from build123d import *

# Parameters (mm, degrees)
F1_DEPTH = 16
F2_W     = 7.5
F2_H     = 58


with BuildPart() as f1:
    # F0 (on Top) → F1 (new body)
    with BuildSketch(Plane.XY):
        with BuildLine():
            Line((-4.2, -8.4), (4.2, -8.4))
            ThreePointArc((4.2, -8.4), (7.028427, -7.228427), (8.2, -4.4))
            Line((8.2, -4.4), (8.2, 4.4))
            ThreePointArc((8.2, 4.4), (7.028427, 7.228427), (4.2, 8.4))
            Line((4.2, 8.4), (-4.2, 8.4))
            ThreePointArc((-4.2, 8.4), (-7.028427, 7.228427), (-8.2, 4.4))
            Line((-8.2, 4.4), (-8.2, -4.4))
            ThreePointArc((-8.2, -4.4), (-7.028427, -7.228427), (-4.2, -8.4))
        make_face()
    extrude(amount=-F1_DEPTH)

    # F2 (on Right) → F3 (revolve)
    with BuildSketch(Plane.YZ):
        Polygon((-10, 0), (0, 0), (0, 1.5), (-7.5, 1.5), (-10, 1.5), align=None)
        with Locations((-3.75, 30.5)):
            Rectangle(F2_W, F2_H)
        Polygon((-7.5, 59.5), (0, 59.5), (0, 60.5), (-8, 60.5), (-8, 59.5), align=None)
    revolve(axis=Axis((0, 0, 30.5), (0, 0, 1)))


solid = f1.part
Source: CAD feature listing. Evaluate the final solid. Frame: model axes, mm. A direction names the side the tool comes from. Coordinates: 2 decimals unless noted, no trailing zeros. Loops run counter-clockwise (first coordinate to the right, second up) from the corner with the lowest first, then second, coordinate; pieces in that order, holes last. Notation, with made-up numbers: M 73.5,34.25 L 113.5,34.25 A27 ccw 113.5,50.25 Z; hole C -25,16 d2. An arc over 180 degrees is marked long. Answer in a Markdown table with one row per item.
Q1. Section B-B on y = 0. Return the cut outline in (x, z), plus the area to 3 significant figures.
Answers below:
| item | result |
|---|---|
| outline | M -10,0 L -8.2,0 L -8.2,-16 L 8.2,-16 L 8.2,0 L 10,0 L 10,1.5 L 7.5,1.5 L 7.5,59.5 L 8,59.5 L 8,60.5 L -8,60.5 L -8,59.5 L -7.5,59.5 L -7.5,1.5 L -10,1.5 Z |
| area | 1,180 mm^2 |
Q2. Draft query along Z for faces 1 (the flat face through (-6, -5, 59.5)), 2 (the flat face through (9, 0, 0)), 3 (the flat face through (0, 0, 60.5)). Return one class per face: pulls with the +Z half, pulls with the -Z half, needs draft (parallel to the pull), parting line crosses it, or undercut.
Answers below:
| item | result |
|---|---|
| face 1 | undercut |
| face 2 | pulls with the -Z half |
| face 3 | pulls with the +Z half |
Q3. First-contact query: pin 1 (1 mm diameter, centred on x = 3, z = 32, fed in from -Y); pin 2 (8 mm diameter, centred on y = 7, z = 41.5, fed in from +X); pin 3 (0.7 mm diameter, centred on x = 7, y = -7.5, fed in from +Z). Flat tips, straight axial feed; report the tip coordinate or a pass-through.
Answers below:
| item | result |
|---|---|
| pin 1 | stops at y = -7.07 |
| pin 2 | stops at x = 6.87 |
| pin 3 | stops at z = 1.5 |
Q4. Section A-A on z = -10.5. Return the cut outline in (x, y).
Answers below:
| item | result |
|---|---|
| outline | M -8.2,-4.4 A4 ccw -4.2,-8.4 L 4.2,-8.4 A4 ccw 8.2,-4.4 L 8.2,4.4 A4 ccw 4.2,8.4 L -4.2,8.4 A4 ccw -8.2,4.4 Z |
Q5. Section C-C on x = 0. Return the cut outline in (y, z).
Answers below:
| item | result |
|---|---|
| outline | M -10,0 L -8.4,0 L -8.4,-16 L 8.4,-16 L 8.4,0 L 10,0 L 10,1.5 L 7.5,1.5 L 7.5,59.5 L 8,59.5 L 8,60.5 L -8,60.5 L -8,59.5 L -7.5,59.5 L -7.5,1.5 L -10,1.5 Z |
Q6. Set-up query: faces 4 (the cylindrical face through (-6.997, 7.259, -7.888)), 5 (the cylindrical face through (0.33, 7.493, 30.906)), 6 (the cylindrical face through (-7.81, 1.73, 59.99)), 7 (the cylindrical face through (-7.059, -7.197, -7.888)). Return all of +Z, -Z, +X, -X, +Y, -Y with unobstructed straight access to the full face (end or side cutting, diameter ignored); none if empty.
Answers below:
| item | result |
|---|---|
| face 4 | -Z, -X, +Y |
| face 5 | none |
| face 6 | +Z |
| face 7 | -Z, -X, -Y |
Q7. Ray query, probe 1 along Z at (x, y) = (-8.25, -3.5); probe 2 along X at (y, z) = (-1, -11); probe 3 along X at (y, z) = (-0.25, 45). Return the intervals inside material, ascending. Write a range as from..to.
Answers below:
| item | result |
|---|---|
| probe 1 | z = 0..1.5 |
| probe 2 | x = -8.2..8.2 |
| probe 3 | x = -7.5..7.5 |
Q8. Section D-D on z = 7.5. Return the cut outline in (x, y).
Answers below:
| item | result |
|---|---|
| outline | C 0,0 d15 |
